Part model, mm, in its own coordinate system. A direction names the side the tool comes from. Round coordinates to 2 decimals unless told otherwise and drop trailing zeros. Order: outer loops, then holes, each group sorted by start corner. A loop starts at its lowest first (then second) coordinate and runs counter-clockwise, first axis right, second up. Notation, with made-up numbers: (7.5, 61) - (52.5, 61) arc R10 ccw to (52.5, 67) - close; hole circle Ø4 at (86.5, 88.25). An arc over 180 degrees is marked (long way). Answer as a JSON object with one key per item and string values.
```python
from build123d import *

# Parameters (mm, degrees)
SKETCH2_R = 4
SKETCH3_R = 3.35


with BuildPart() as part:
    # Sweep1: sweep along a path in Sketch1
    with BuildLine(Plane(origin=(0, 0, 0), x_dir=(0, 0, -1), z_dir=(1, 0, 0))) as sweep1_path:
        Line((0, 0), (60, 0))
        ThreePointArc((60, 0), (82.627416998, 9.372583002), (92, 32))
        Line((92, 32), (92, 72))
    # Sketch2 → Sweep1 (sweep)
    with BuildSketch(Plane.XY):
        Circle(SKETCH2_R)
    sweep(path=sweep1_path.line)

    # Cut-Sweep1: sweep along a path in Sketch1<4>
    with BuildLine(Plane(origin=(0, 0, 0), x_dir=(0, 0, -1), z_dir=(1, 0, 0))) as cut_sweep1_path:
        Line((0, 0), (60, 0))
        ThreePointArc((60, 0), (82.627416998, 9.372583002), (92, 32))
        Line((92, 32), (92, 72))
    # Sketch3 → Cut-Sweep1 (sweep, cut)
    with BuildSketch(Plane.XY):
        Circle(SKETCH3_R)
    sweep(path=cut_sweep1_path.line, mode=Mode.SUBTRACT)


solid = part.part
```
Item 1: Cut at A-A (x = 0). Write the cut outline in (y, z), plus the area to 3 significant figures.
Taken from the geometry:
{"outline": "(-4, -60) arc R36 ccw to (32, -96) - (72, -96) - (72, -95.35) - (32, -95.35) arc R35.35 cw to (-3.35, -60) - (-3.35, 0) - (-4, 0) - close; (3.35, -60) arc R28.65 ccw to (32, -88.65) - (72, -88.65) - (72, -88) - (32, -88) arc R28 cw to (4, -60) - (4, 0) - (3.35, 0) - close", "area": "195 mm2"}
Item 2: Drop flat-ended pins along their axis: P1, Ø4, axis at x = -3, z = -27, coming from the -Y side; P2, Ø4, axis at x = 2, y = 17, coming from the -Z side; P3, Ø4, axis at x = 0, z = -47.5, coming from the +Y side. Give the stop position or say it passes through.
Taken from the geometry:
{"P1": "y = -3.87", "P2": "z = -93.33", "P3": "y = 4"}
Item 3: Two-plate mould, pull along X, no slides. Class faces 1 (the flat face through (2, -3, 0)), 2 (the cylindrical face through (1.846, 52.28, -88.451)), 3 (the cylindrical face through (-3.347, -0.147, -30.42)), 4 (the cylindrical face through (-0.44, 52.28, -95.32)): pulls with the +X half, pulls with the -X half, needs draft (parallel to the pull), parting line crosses it, or undercut.
Taken from the geometry:
{"face 1": "needs draft", "face 2": "parting line crosses it", "face 3": "undercut", "face 4": "undercut"}
Item 4: Cut at C-C (y = 49). Write the cut outline in (x, z), plus the area to 3 significant figures.
Taken from the geometry:
{"outline": "circle Ø8 at (0, -92); hole circle Ø6.7 at (0, -92)", "area": "15.0 mm2"}
Item 5: Probe L1, parallel to X at y = 0, z = -25.5; L2, parallel to Z at x = 0, y = 53; L3, parallel to Y at x = -0.25, z = -5. List the from-to ranges inside material, lowest first. Write a range as from..to.
Taken from the geometry:
{"L1": "-4..-3.35, 3.35..4", "L2": "-96..-95.35, -88.65..-88", "L3": "-3.99..-3.34, 3.34..3.99"}
Item 6: Cut at B-B (z = -57). Write the cut outline in (x, y), plus the area to 3 significant figures.
Taken from the geometry:
{"outline": "circle Ø8 at (0, 0); hole circle Ø6.7 at (0, 0)", "area": "15.0 mm2"}
Item 7: Tool access for faces 5 (the cylindrical face through (-0.867, 3.905, -30.42)), 6 (the flat face through (-3, 72, -94)): list every direction of +Z, -Z, +X, -X, +Y, -Y with a clear straight run to the whole face (end or side of a thin tool).
Taken from the geometry:
{"face 5": "+Z", "face 6": "+Z, -Z, +X, -X, +Y"}
